Can you work these out from the model? Positions are in its coordinate system, mm. A direction names the side the tool comes from. Give positions to 0.01 mm unless a question says otherwise; leave off trailing zeros. Loops run counter-clockwise (first coordinate to the right, second up) from the corner with the lowest first, then second, coordinate; pieces in that order, holes last. Notation, with made-up numbers: (43.5, 57.5) - (98.5, 57.5) arc R10 ccw to (98.5, 62.5) - close; hole circle Ø1 at (-38.5, -17.75). An arc over 180 degrees is marked (long way). Answer as a JSON object with one key per item and string values. Group by question number.
Item 1: Suppose I cut it at B-B on z = 5. Write out the boundary of the cut face in (x, y).
Item 2: Which directions (+Z, -Z, +X, -X, +Y, -Y) give clear straight access to the entire face, cutting with the end or side of a thin tool? Please do faces 1 (the cylindrical face through (59.526, -12.148, 9.584)), 2 (the flat face through (91, -19, 7.1)).
Item 3: Thinking about a two-plate mould opening in X: for faces 3 (the flat face through (180, -19, 6)), 4 (the flat face through (89, 0, 9)), 5 (the flat face through (164, -19, 4)), which applies, pulls with the +X half, pulls with the -X half, needs draft (parallel to the pull), parting line crosses it, or undercut?
Item 4: Suppose I cut it at D-D on y = -19.5. Write out the boundary of the cut face in (x, z).
Item 5: Suppose I cut it at A-A on x = 151. Write out the boundary of the cut face in (y, z), and give its area (3 significant figures).
Item 6: Please list where these lines run through material, in increasing order: L1, parallel to Y at x = 119, z = 10.9; L2, parallel to Y at x = 170, z = 4; L3, parallel to X at y = -26.5, z = 4.
Item 7: Suppose I cut it at C-C on x = 170. Write out the boundary of the cut face in (y, z).
Item 8: Will these pins go through, and if not, where does the flat tip stop? pin 1 (4.5 mm diameter, centred on x = 119, y = -13.5, fed in from -Z); pin 2 (1 mm diameter, centred on x = 18, z = 10, fed in from +Y).
from build123d import *

# Parameters (mm, degrees)
SKETCH1_W           = 180
SKETCH1_H           = 38
SKETCH1_R           = 2.35
BOSS_EXTRUDE1_DEPTH = 12
CUT_EXTRUDE1_DEPTH  = 38
SKETCH3_R           = 2
CUT_EXTRUDE2_DEPTH  = 22


with BuildPart() as part:
    # Sketch1 → Boss-Extrude1 (new body)
    with BuildSketch(Plane.XY):
        with Locations((90, -19)):
            Rectangle(SKETCH1_W, SKETCH1_H)
        with Locations((170, -10)):
            Circle(SKETCH1_R, mode=Mode.SUBTRACT)
        with Locations((170, -27.996930787)):
            Circle(SKETCH1_R, mode=Mode.SUBTRACT)
        with Locations((10, -10)):
            Circle(SKETCH1_R, mode=Mode.SUBTRACT)
        with Locations((10, -27.996930787)):
            Circle(SKETCH1_R, mode=Mode.SUBTRACT)
    extrude(amount=BOSS_EXTRUDE1_DEPTH)

    # Sketch2 → Cut-Extrude1 (cut)
    with BuildSketch(Plane(origin=(0, 0, 0), x_dir=(1, 0, 0), z_dir=(0, 1, 0))):
        Polygon((168, 0), (160.9, -7.1), (19.1, -7.1), (12, 0), align=None)
    extrude(amount=-CUT_EXTRUDE1_DEPTH, mode=Mode.SUBTRACT)

    # Sketch3 → Cut-Extrude2 (cut)
    with BuildSketch(Plane.XY.offset(12)):
        with Locations((151, -13.5)):
            Circle(SKETCH3_R)
        with Locations((119, -13.5)):
            Circle(SKETCH3_R)
        with Locations((106, -13.5)):
            Circle(SKETCH3_R)
        with Locations((74, -13.5)):
            Circle(SKETCH3_R)
        with Locations((61, -13.5)):
            Circle(SKETCH3_R)
        with Locations((29, -13.5)):
            Circle(SKETCH3_R)
    extrude(amount=-CUT_EXTRUDE2_DEPTH, mode=Mode.SUBTRACT)


solid = part.part
Worked out:
{
 "1": {"outline": "(0, -38) - (17, -38) - (17, 0) - (0, 0) - close; (163, -38) - (180, -38) - (180, 0) - (163, 0) - close; hole circle Ø4.7 at (10, -28); hole circle Ø4.7 at (10, -10); hole circle Ø4.7 at (170, -28); hole circle Ø4.7 at (170, -10)"},
 "2": {"face 1": "+Z, -Z", "face 2": "-Z, +Y, -Y"},
 "3": {"face 3": "pulls with the +X half", "face 4": "needs draft", "face 5": "undercut"},
 "4": {"outline": "(0, 0) - (12, 0) - (19.1, 7.1) - (160.9, 7.1) - (168, 0) - (180, 0) - (180, 12) - (0, 12) - close"},
 "5": {"outline": "(-38, 7.1) - (-15.5, 7.1) - (-15.5, 12) - (-38, 12) - close; (-11.5, 7.1) - (0, 7.1) - (0, 12) - (-11.5, 12) - close", "area": "167 mm2"},
 "6": {"L1": "y = -38 to -15.5, -11.5 to 0", "L2": "y = -38 to -30.35, -25.65 to -12.35, -7.65 to 0", "L3": "x = 0 to 8.19, 11.81 to 16, 164 to 168.19, 171.81 to 180"},
 "7": {"outline": "(-38, 0) - (-30.35, 0) - (-30.35, 12) - (-38, 12) - close; (-25.65, 0) - (-12.35, 0) - (-12.35, 12) - (-25.65, 12) - close; (-7.65, 0) - (0, 0) - (0, 12) - (-7.65, 12) - close"},
 "8": {"pin 1": "stops at z = 7.1", "pin 2": "stops at y = 0"}
}
